from build123d import *

# Parameters (mm, degrees)
F1_DEPTH = 4
F2_R     = 2
F3_R     = 1.99999


# Not quite as in the source:
# - a fillet or chamfer is up to 0.001 mm smaller than in the source, because OpenCascade refuses the exact size


with BuildPart() as f1:
    # F0 (on Top) → F1 (new body)
    with BuildSketch(Plane.XY):
        Polygon((-82.9944183651, 27.933470586), (-90.9944183651, 35.933470586), (-102.3081268641, 35.933470586), (-31.5974487455, -34.7772075326), (-31.5974487455, -23.4634990336), (-37.5931606391, -17.46778714), (-60.9944183651, 5.933470586), (-62.9944183651, 7.933470586), (-70.9944183651, 15.933470586), (-72.9944183651, 17.933470586), (-80.9944183651, 25.933470586), align=None)
        with BuildLine():
            Line((-60.9944183651, 5.933470586), (-37.5931606391, -17.46778714))
            ThreePointArc((-37.5931606391, -17.46778714), (-39.4312238538, -8.2272193518), (-31.5974487455, -2.9928581702))
            Line((-31.5974487455, -2.9928581702), (-31.5974487455, 5.933470586))
            Line((-31.5974487455, 5.933470586), (-60.9944183651, 5.933470586))
        make_face()
        with BuildLine():
            Line((-31.5974487455, -19.9512923224), (-31.5974487455, -23.4634990336))
            Line((-31.5974487455, -23.4634990336), (-25.6017368518, -17.46778714))
            ThreePointArc((-25.6017368518, -17.46778714), (-28.352592851, -19.3058503546), (-31.5974487455, -19.9512923224))
        make_face()
        Polygon((39.1132293732, 35.933470586), (27.7995208742, 35.933470586), (19.7995208742, 27.933470586), (17.7995208742, 25.933470586), (9.7995208742, 17.933470586), (7.7995208742, 15.933470586), (-0.2004791258, 7.933470586), (-2.2004791258, 5.933470586), (-25.6017368518, -17.46778714), (-31.5974487455, -23.4634990336), (-31.5974487455, -34.7772075326), align=None)
        with BuildLine():
            Line((-37.5931606391, -17.46778714), (-31.5974487455, -23.4634990336))
            Line((-31.5974487455, -23.4634990336), (-31.5974487455, -19.9512923224))
            ThreePointArc((-31.5974487455, -19.9512923224), (-34.8423046399, -19.3058503546), (-37.5931606391, -17.46778714))
        make_face()
        with BuildLine():
            ThreePointArc((-23.1182316693, -11.4720752463), (-23.7636736371, -14.7169311407), (-25.6017368518, -17.46778714))
            Line((-25.6017368518, -17.46778714), (-2.2004791258, 5.933470586))
            Line((-2.2004791258, 5.933470586), (-31.5974487455, 5.933470586))
            Line((-31.5974487455, 5.933470586), (-31.5974487455, -2.9928581702))
            ThreePointArc((-31.5974487455, -2.9928581702), (-25.6017368518, -5.4763633526), (-23.1182316693, -11.4720752463))
        make_face()
        Polygon((7.7995208742, 15.933470586), (-31.5974487455, 15.933470586), (-31.5974487455, 7.933470586), (-0.2004791258, 7.933470586), align=None)
        Polygon((-31.5974487455, 7.933470586), (-31.5974487455, 15.933470586), (-70.9944183651, 15.933470586), (-62.9944183651, 7.933470586), align=None)
        Polygon((17.7995208742, 25.933470586), (-31.5974487455, 25.933470586), (-31.5974487455, 17.933470586), (9.7995208742, 17.933470586), align=None)
        Polygon((-31.5974487455, 17.933470586), (-31.5974487455, 25.933470586), (-80.9944183651, 25.933470586), (-72.9944183651, 17.933470586), align=None)
        Polygon((27.7995208742, 35.933470586), (-31.5974487455, 35.933470586), (-31.5974487455, 27.933470586), (19.7995208742, 27.933470586), align=None)
        Polygon((-31.5974487455, 27.933470586), (-31.5974487455, 35.933470586), (-90.9944183651, 35.933470586), (-82.9944183651, 27.933470586), align=None)
    extrude(amount=F1_DEPTH)

    # F2
    f2_edges = [f1.edges().sort_by_distance(p)[0] for p in [
        (-31.597449, 35.933471, 4),
        (-31.597449, 27.933471, 4),
        (-31.597449, 25.933471, 4),
        (-31.597449, 17.933471, 4),
        (-31.597449, 15.933471, 4),
        (-31.597449, 7.933471, 4),
        (-31.597449, 5.933471, 4),
        (-66.952788, 0.578132, 4),
        (3.75789, 0.578132, 4),
        (8.799521, 16.933471, 4),
        (18.799521, 26.933471, 4),
        (-1.200479, 6.933471, 4),
        (-61.994418, 6.933471, 4),
        (-71.994418, 16.933471, 4),
        (-81.994418, 26.933471, 4),
    ]]
    fillet(f2_edges, radius=F2_R)

    # F3 (radius 2 in the source; OpenCascade refuses exactly that, so slightly less here)
    f3_edges = [f1.edges().sort_by_distance(p)[0] for p in [
        (-31.597449, 27.933471, 0),
        (-31.597449, 25.933471, 0),
        (-31.597449, 7.933471, 0),
        (-31.597449, 5.933471, 0),
        (-31.597449, 17.933471, 0),
        (-31.597449, 15.933471, 0),
    ]]
    fillet(f3_edges, radius=F3_R)


solid = f1.part
Source: CAD feature listing. Evaluate the final solid. Frame: model axes, mm. Round coordinates to 2 decimals unless told otherwise and drop trailing zeros. Loops run counter-clockwise (first coordinate to the right, second up) from the corner with the lowest first, then second, coordinate; pieces in that order, holes last. Notation, with made-up numbers: M -35.75,32 L 11.25,32 A32 ccw 11.25,68 Z; hole C -19,-14.75 d11. An arc over 180 degrees is marked long. Return JSON: item names as keys, results as strings. Group by question number.
1. Material intervals for line 1 along Y through (x, z) = (7.5, 2.4); line 2 along Y through (x, z) = (-39, 0.6); line 3 along Y through (x, z) = (8.5, 1.2), sorted ascending. Write a range as from..to.
2. Section query B-B on x = -35.5. State how many separate pieces and enclosed holes the cut face has, and give its area (3 significant figures).
3. Mould query, pull axis X, two halves, no side actions, for faces 1 (the face through (20.095, 27.049, 3.626)), 2 (the face through (-1.158, 6.975, 0.764)), 3 (the face through (-32, 21, 4)), 4 (the face through (-67.448, 1.073, 0.986)). Classes: released by +X, released by -X, zero draft, split by the parting line, or undercut.
4. Section query A-A on z = 1.3. Output: boundary loops of the cut face in (x, y).
Checks:
{
 "1": {"line 1": "y = 4.38..15.89, 17.97..25.89, 27.97..35.89", "line 2": "y = -27.37..-15.61, -7.34..5.36, 8.51..15.36, 18.51..25.36, 28.51..35.93", "line 3": "y = 5.32..16.63, 18.1..25.77, 28.1..35.93"},
 "2": {"separate pieces": "5", "enclosed holes": "0", "area": "171 mm²"},
 "3": {"face 1": "undercut", "face 2": "undercut", "face 3": "zero draft", "face 4": "released by -X"},
 "4": {"outline": "M -102.31,35.93 L -31.6,-34.78 L 39.11,35.93 Z; hole M -83.12,28.06 L -80.87,25.81 L 17.67,25.81 L 19.93,28.06 Z; hole M -73.12,18.06 L -70.87,15.81 L 7.67,15.81 L 9.93,18.06 Z; hole M -63.12,8.06 L -60.87,5.81 L -2.33,5.81 L -0.07,8.06 Z; hole C -31.6,-11.47 d16.96"}
}
